Source: CAD feature listing. Evaluate the final solid. Frame: model axes, mm. A direction names the side the tool comes from. Give positions to 0.01 mm unless a question says otherwise; leave off trailing zeros. Loops run counter-clockwise (first coordinate to the right, second up) from the corner with the lowest first, then second, coordinate; pieces in that order, holes last. Notation, with made-up numbers: M -15.75,-19.75 L 24.25,-19.75 A17 ccw 24.25,-3.75 Z; hole C 41.25,-19 d5. An arc over 180 degrees is marked long. Put each result on its own line as item: value.
from build123d import *

# Parameters (mm, degrees)
F0_W     = 47
F0_H     = 61
F0_R     = 2.75
F1_DEPTH = 8


with BuildPart() as f1:
    # F0 (on Front) → F1 (new body)
    with BuildSketch(Plane.XZ):
        Rectangle(F0_W, F0_H)
        with Locations((-12.5, -24.5)):
            Circle(F0_R, mode=Mode.SUBTRACT)
        with Locations((12.5, -24.5)):
            Circle(F0_R, mode=Mode.SUBTRACT)
        with Locations((-12.5, 10.5)):
            Circle(F0_R, mode=Mode.SUBTRACT)
        with BuildLine():
            ThreePointArc((-14.900004, 24.504627), (-17.504354, 21.900004), (-20.099966, 24.513334))
            Line((-20.099966, 24.513334), (-20.1, 26.499955))
            ThreePointArc((-20.1, 26.499955), (-17.434316, 29.09917), (-14.903321, 26.368629))
            Line((-14.903321, 26.368629), (-14.900004, 24.504627))
        make_face(mode=Mode.SUBTRACT)
        with Locations((12.5, 10.5)):
            Circle(F0_R, mode=Mode.SUBTRACT)
        with BuildLine():
            Line((20.1, 26.499955), (20.099966, 24.513334))
            ThreePointArc((20.099966, 24.513334), (17.504354, 21.900004), (14.900004, 24.504627))
            Line((14.900004, 24.504627), (14.903321, 26.368629))
            ThreePointArc((14.903321, 26.368629), (17.434316, 29.09917), (20.1, 26.499955))
        make_face(mode=Mode.SUBTRACT)
    extrude(amount=F1_DEPTH)


solid = f1.part
1. Section query A-A (x = -17.5). Output: boundary loops of the cut face in (y, z).
Found:
outline: M -8,-30.5 L 0,-30.5 L 0,21.9 L -8,21.9 Z; M -8,29.1 L 0,29.1 L 0,30.5 L -8,30.5 Z
2. Access query for faces 1 (the cylindrical face through (-17.5, -3.9, 29.1)), 2 (the flat face through (-23.5, -4, 0)). Directions: +Z, -Z, +X, -X, +Y, -Y. A direction counts if a zero-diameter tool reaches every point of the face in a straight line with its end or side. Return the directions, or none.
Found:
face 1: +Y, -Y
face 2: +Z, -Z, -X, +Y, -Y
3. Section query D-D (z = 10.5). Output: boundary loops of the cut face in (x, y).
Found:
outline: M -23.5,-8 L -15.25,-8 L -15.25,0 L -23.5,0 Z; M -9.75,-8 L 9.75,-8 L 9.75,0 L -9.75,0 Z; M 15.25,-8 L 23.5,-8 L 23.5,0 L 15.25,0 Z
4. Material intervals for line 1 (Z direction, x = -12.5, y = -4); line 2 (X direction, y = -5.25, z = 12.5); line 3 (Z direction, x = 11.5, y = -0.25), sorted ascending. Write a range as from..to.
Found:
line 1: -30.5..-27.25, -21.75..7.75, 13.25..30.5
line 2: -23.5..-14.39, -10.61..10.61, 14.39..23.5
line 3: -30.5..-27.06, -21.94..7.94, 13.06..30.5
5. Draft query along X for faces 3 (the flat face through (23.5, -4, 0)), 4 (the flat face through (0, 0, 0)), 5 (the cylindrical face through (17.4, -3.9, 29.1)), 6 (the cylindrical face through (17.6, -3.9, 21.9)). Return one class per face: pulls with the +X half, pulls with the -X half, needs draft (parallel to the pull), parting line crosses it, or undercut.
Found:
face 3: pulls with the +X half
face 4: needs draft
face 5: undercut
face 6: undercut
6. Section query B-B (y = -5.5). Output: boundary loops of the cut face in (x, z).
Found:
outline: M -23.5,-30.5 L 23.5,-30.5 L 23.5,30.5 L -23.5,30.5 Z; hole M -20.1,24.51 A2.6 ccw long -14.9,24.5 L -14.9,26.37 A2.6 ccw long -20.1,26.5 Z; hole C -12.5,-24.5 d5.5; hole C -12.5,10.5 d5.5; hole C 12.5,-24.5 d5.5; hole C 12.5,10.5 d5.5; hole M 14.9,24.5 A2.6 ccw long 20.1,24.51 L 20.1,26.5 A2.6 ccw long 14.9,26.37 Z
7. Section query C-C (x = 12.5). Output: boundary loops of the cut face in (y, z).
Found:
outline: M -8,-30.5 L 0,-30.5 L 0,-27.25 L -8,-27.25 Z; M -8,-21.75 L 0,-21.75 L 0,7.75 L -8,7.75 Z; M -8,13.25 L 0,13.25 L 0,30.5 L -8,30.5 Z
